```python
from build123d import *

# Parameters (mm, degrees)
SKETCH1_R               = 12
SKETCH1_R_2             = 0.5
SKETCH1_R_3             = 6
BOSS_EXTRUDE1_DEPTH     = 1.5
SKETCH6_W               = 0.8
SKETCH6_H               = 0.5
CUT_EXTRUDE1_DEPTH      = 19.163975336
CUT_EXTRUDE1_DEPTH_BACK = 19.163975336
CUT_EXTRUDE2_DEPTH      = 19.348841925
CUT_EXTRUDE2_DEPTH_BACK = 19.348841925
SKETCH5_R               = 0.5
SKETCH5_R_2             = 0.48729794
FILLET1_R               = 0.5
FILLET2_R               = 1


with BuildPart() as part:
    # Sketch1 → Boss-Extrude1 (new, symmetric)
    with BuildSketch(Plane.XY):
        Circle(SKETCH1_R)
        with Locations((9.6, 0)):
            Circle(SKETCH1_R_2, mode=Mode.SUBTRACT)
        Circle(SKETCH1_R_3, mode=Mode.SUBTRACT)
        with Locations((0, -9.6)):
            Circle(SKETCH1_R_2, mode=Mode.SUBTRACT)
        with Locations((-9.6, 0)):
            Circle(SKETCH1_R_2, mode=Mode.SUBTRACT)
        with Locations((0, 9.6)):
            Circle(SKETCH1_R_2, mode=Mode.SUBTRACT)
    extrude(amount=BOSS_EXTRUDE1_DEPTH, both=True)

    # Sketch2 → Cut-Revolve1 (revolve, cut)
    with BuildSketch(Plane(origin=(0, 0, 0), x_dir=(1, 0, 0), z_dir=(0, 1, 0)), mode=Mode.PRIVATE) as cut_revolve1_sk:
        with BuildLine():
            Line((-11.5, 0.5), (-11.5, -0.5))
            ThreePointArc((-11.5, -0.5), (-11.646446609, -0.853553391), (-12, -1))
            Line((-12, -1), (-12, 1))
            ThreePointArc((-12, 1), (-11.646446609, 0.853553391), (-11.5, 0.5))
        make_face()
    revolve(cut_revolve1_sk.sketch.rotate(Axis((0, 0, 0), (0, 0, -1)), 180), axis=Axis((0, 0, 0), (0, 0, -1)), mode=Mode.SUBTRACT)

    # Sketch6 → Revolve1 (revolve)
    with BuildSketch(Plane(origin=(0, 0, 0), x_dir=(1, 0, 0), z_dir=(0, 1, 0))):
        with Locations((12.4, 1.25)):
            Rectangle(SKETCH6_W, SKETCH6_H)
        with Locations((12.4, -1.25)):
            Rectangle(SKETCH6_W, SKETCH6_H)
    revolve(axis=Axis((0, 0, 0), (0, 0, -1)))

    # Sketch4 → Cut-Extrude1 (cut, two sides: drawn at the far end of the back side and taken through both)
    with BuildSketch(Plane.XY.offset(-CUT_EXTRUDE1_DEPTH_BACK)):
        Polygon((-3.743635752, 13.97143883), (0, 0), (14.900233226, -3.99250546), (14.900233226, -14.839385646), (-15.188066433, -14.839385646), (-15.188066433, 13.97143883), align=None)
    extrude(amount=CUT_EXTRUDE1_DEPTH + CUT_EXTRUDE1_DEPTH_BACK, mode=Mode.SUBTRACT)

    # Sketch5 → Cut-Extrude2 (cut, two sides: drawn at the far end of the back side and taken through both)
    with BuildSketch(Plane.XY.offset(1.5).offset(-CUT_EXTRUDE2_DEPTH_BACK)):
        with Locations((-2.67687174, 9.990221337)):
            Circle(SKETCH5_R)
        with Locations((-1.026834566, 10.829057404)):
            Circle(SKETCH5_R_2)
    extrude(amount=CUT_EXTRUDE2_DEPTH + CUT_EXTRUDE2_DEPTH_BACK, mode=Mode.SUBTRACT)

    # Fillet1
    fillet1_edges = [part.edges().sort_by_distance(p)[0] for p in [
        (4.242640687, 4.242640687, 1.5),
        (4.242640687, 4.242640687, -1.5),
    ]]
    fillet(fillet1_edges, radius=FILLET1_R)

    # Fillet2
    fillet2_edges = [part.edges().sort_by_distance(p)[0] for p in [
        (12.363850577, -3.312883777, -1.25),
        (12.363850577, -3.312883777, 1.25),
        (-3.312883777, 12.363850577, -1.25),
        (-3.312883777, 12.363850577, 1.25),
    ]]
    fillet(fillet2_edges, radius=FILLET2_R)


solid = part.part
```
Verification items for the finished model (mm, model axes). Give positions to 0.01 mm unless a question says otherwise; leave off trailing zeros. Order: outer loops, then holes, each group sorted by start corner. A loop starts at its lowest first (then second) coordinate and runs counter-clockwise, first axis right, second up. Notation, with made-up numbers: M 54,61 L 84,61 A20 cw 84,87 Z; hole C 40.5,64 d4. An arc over 180 degrees is marked long. Return JSON: item names as keys, results as strings. Group by question number.
1) Go/stop test with flat-tipped pins: pin 1 Ø1.5 at (x, z) = (-1, 1) entering from -Y; pin 2 Ø2 at (x, y) = (4, 0) entering from +Z; pin 3 Ø1 at (y, z) = (11, 0) entering from -X. Record where each tip stops, or that it passes through.
2) Scan lines: line 1 (Z direction, x = 6, y = 10.5); line 2 (Y direction, x = 9.6, z = -0.3); line 3 (Y direction, x = 9.6, z = 0.65). Record each from-to range of solid material in increasing order.
3) Mould release check, pull along Z, two halves, no side actions. Record for faces 1 (the face through (9, 8.4, 1)), 2 (the face through (9, 8.4, -1)), 3 (the face through (0.231, 9.156, -0.021)), 4 (the face through (7, 5, 1.5)): pulls with the +Z half, pulls with the -Z half, needs draft (parallel to the pull), parting line crosses it, or undercut.
4) Section check A-A on y = 0. Record the cut outline in (x, z), and give its area (3 significant figures).
Answer block:
{
 "1": {"pin 1": "stops at y = 5.8", "pin 2": "passes through", "pin 3": "stops at x = -2.98"},
 "2": {"line 1": "z = -1.5 to -1, 1 to 1.5", "line 2": "y = -2.57 to -0.5, 0.5 to 6.33", "line 3": "y = -2.57 to -0.5, 0.5 to 6.37"},
 "3": {"face 1": "undercut", "face 2": "undercut", "face 3": "needs draft", "face 4": "pulls with the +Z half"},
 "4": {"outline": "M 6,-1 A0.5 ccw 6.5,-1.5 L 9.1,-1.5 L 9.1,1.5 L 6.5,1.5 A0.5 ccw 6,1 Z; M 10.1,-1.5 L 12.8,-1.5 L 12.8,-1 L 12,-1 A0.5 cw 11.5,-0.5 L 11.5,0.5 A0.5 cw 12,1 L 12.8,1 L 12.8,1.5 L 10.1,1.5 Z", "area": "14.8 mm^2"}
}
